The model under review builds one solid part; all positions refer to its coordinate system, in mm. Round coordinates to 2 decimals unless told otherwise and drop trailing zeros. Order: outer loops, then holes, each group sorted by start corner. A loop starts at its lowest first (then second) coordinate and runs counter-clockwise, first axis right, second up. Notation, with made-up numbers: M 88,2.5 L 93,2.5 A21 ccw 93,29.5 Z; hole C 70.5,-36.75 d4. An arc over 180 degrees is marked long. Answer as a JSON object with one key per item and string values. Group by question number.
1) To check wall thickness, follow line 1 (X direction, y = -0.4, z = 25.4); line 2 (Z direction, x = -368.3, y = -0.8); line 3 (X direction, y = 0.95, z = -343.5). State the ranges of each line that lie inside material, in increasing order.
2) Insertion check: pin 1 Ø1 at (x, y) = (-312.5, 0) entering from +Z; pin 2 Ø4 at (x, z) = (327.025, 0) entering from +Y; pin 3 Ø1.6 at (y, z) = (0, 350) entering from -X; pin 4 Ø1.6 at (x, y) = (-344.5, 0) entering from -Z. Each pin has a flat end and moves straight along its axis. Give the tip position at first contact, or say it passes through.
3) Consider section A-A, the plane y = 0.7. Count the separate pieces of the cut face and the enclosed holes in it, then the cut area to 3 significant figures.
4) Consider section C-C, the plane z = 235. Write out the cut boundary in (x, y).
5) Consider section B-B, the plane x = -309.5. Write out the cut boundary in (y, z).
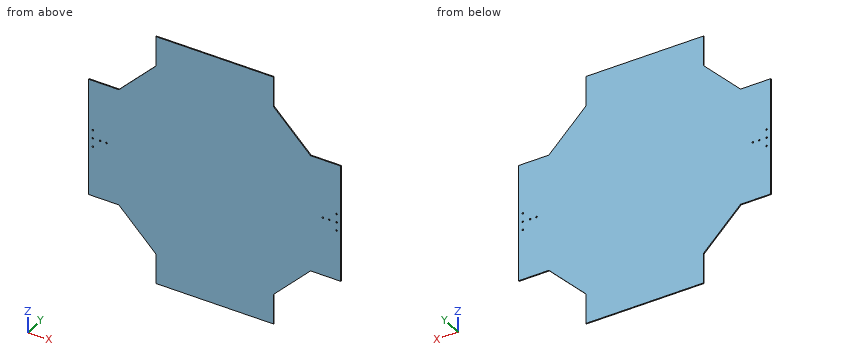
```python
from build123d import *

# Parameters (mm, degrees)
BOSS_EXTRUDE1_DEPTH = 1.5875
SKETCH2_R           = 2.38125
CUT_EXTRUDE1_DEPTH  = 539.824721616


with BuildPart() as part:
    # Sketch1 → Boss-Extrude1 (new, symmetric)
    with BuildSketch(Plane(origin=(0, 0, 0), x_dir=(1, 0, 0), z_dir=(0, 1, 0))):
        Polygon((-381, 177.8), (-289.71875, 177.8), (-177.8, 289.71875), (-177.8, 381), (177.8, 381), (177.8, 289.71875), (289.71875, 177.8), (381, 177.8), (381, -177.8), (289.71875, -177.8), (177.8, -289.71875), (177.8, -381), (-177.8, -381), (-177.8, -289.71875), (-289.71875, -177.8), (-381, -177.8), align=None)
    extrude(amount=BOSS_EXTRUDE1_DEPTH, both=True)

    # Sketch2 → Cut-Extrude1 (cut, through all)
    with BuildSketch(Plane(origin=(0, 1.5875, 0), x_dir=(1, 0, 0), z_dir=(0, 1, 0))):
        with Locations(Location((-346.075, 0, 0), (0, 0, 270))):
            Circle(SKETCH2_R)
        with Locations(Location((-368.3, 0, 0), (0, 0, 270))):
            Circle(SKETCH2_R)
        with Locations(Location((-368.3, 25.4, 0), (0, 0, 270))):
            Circle(SKETCH2_R)
        with Locations(Location((-368.3, -25.4, 0), (0, 0, 270))):
            Circle(SKETCH2_R)
        with Locations(Location((368.3, -25.4, 0), (0, 0, 90))):
            Circle(SKETCH2_R)
        with Locations(Location((368.3, 25.4, 0), (0, 0, 90))):
            Circle(SKETCH2_R)
        with Locations(Location((368.3, 0, 0), (0, 0, 90))):
            Circle(SKETCH2_R)
        with Locations(Location((346.075, 0, 0), (0, 0, 90))):
            Circle(SKETCH2_R)
        with Locations(Location((-327.025, 0, 0), (0, 0, 270))):
            Circle(SKETCH2_R)
        with Locations(Location((327.025, 0, 0), (0, 0, 270))):
            Circle(SKETCH2_R)
    extrude(amount=-CUT_EXTRUDE1_DEPTH, mode=Mode.SUBTRACT)


solid = part.part
```
Results list:
{
 "1": {"line 1": "-381 to -370.68, -365.92 to 365.92, 370.68 to 381", "line 2": "-177.8 to -27.78, -23.02 to -2.38, 2.38 to 23.02, 27.78 to 177.8", "line 3": "-177.8 to 177.8"},
 "2": {"pin 1": "z = 177.8", "pin 2": "through", "pin 3": "x = -177.8", "pin 4": "z = -177.8"},
 "3": {"separate pieces": "1", "enclosed holes": "10", "area": "440,000 mm^2"},
 "4": {"outline": "M -232.52,-1.59 L 232.52,-1.59 L 232.52,1.59 L -232.52,1.59 Z"},
 "5": {"outline": "M -1.59,-177.8 L 1.59,-177.8 L 1.59,177.8 L -1.59,177.8 Z"}
}
